Check sheet for the modelled part. Datum: model origin and axes. Units: mm. A direction names the side the tool comes from. Give positions to 0.01 mm unless a question says otherwise; leave off trailing zeros. Order: outer loops, then holes, each group sorted by start corner. A loop starts at its lowest first (then second) coordinate and runs counter-clockwise, first axis right, second up. Notation, with made-up numbers: M 63,28 L 97,28 A29 ccw 97,49 Z; hole C 79,15 d6. An arc over 180 degrees is marked long. One line per question, with ' | ' between items. Start each with the question number.
```python
from build123d import *

# Parameters (mm, degrees)
F1_DEPTH = 2
F2_R     = 2
F3_R     = 0.5


with BuildPart() as f1:
    # F0 (on Top) → F1 (new body)
    with BuildSketch(Plane.XY):
        with BuildLine():
            Line((2.5, 7.5), (2.5, 0))
            ThreePointArc((2.5, 0), (0, -2.5), (-2.5, 0))
            Line((-2.5, 0), (-2.5, 7.5))
            Line((-2.5, 7.5), (-7.5, 7.5))
            Line((-7.5, 7.5), (-7.5, -7.5))
            Line((-7.5, -7.5), (7.5, -7.5))
            Line((7.5, -7.5), (7.5, 7.5))
            Line((7.5, 7.5), (2.5, 7.5))
        make_face()
    extrude(amount=F1_DEPTH)

    # F2
    f2_edges = [f1.edges().sort_by_distance(p)[0] for p in [
        (7.5, -7.5, 1),
        (-7.5, -7.5, 1),
        (7.5, 7.5, 1),
        (2.5, 7.5, 1),
        (-2.5, 7.5, 1),
        (-7.5, 7.5, 1),
    ]]
    fillet(f2_edges, radius=F2_R)

    # F3
    f3_edges = [f1.edges().sort_by_distance(p)[0] for p in [
        (7.5, 0, 2),
        (6.914214, -6.914214, 2),
        (6.914214, 6.914214, 2),
        (0, -7.5, 2),
        (5, 7.5, 2),
        (-6.914214, -6.914214, 2),
        (3.085786, 6.914214, 2),
        (-7.5, 0, 2),
        (2.5, 2.75, 2),
        (-6.914214, 6.914214, 2),
        (0, -2.5, 2),
        (-5, 7.5, 2),
        (-2.5, 2.75, 2),
        (-3.085786, 6.914214, 2),
        (7.5, 0, 0),
        (6.914214, -6.914214, 0),
        (6.914214, 6.914214, 0),
        (0, -7.5, 0),
        (5, 7.5, 0),
        (-6.914214, -6.914214, 0),
        (3.085786, 6.914214, 0),
        (-7.5, 0, 0),
        (2.5, 2.75, 0),
        (-6.914214, 6.914214, 0),
        (0, -2.5, 0),
        (-5, 7.5, 0),
        (-2.5, 2.75, 0),
        (-3.085786, 6.914214, 0),
    ]]
    fillet(f3_edges, radius=F3_R)


solid = f1.part
```
Item 1: Section check A-A, the plane y = 3.75. Record the cut outline in (x, z), then the cut area to 3 significant figures.
Item 2: Scan lines: probe 1 along X at (y, z) = (3, 1.2); probe 2 along X at (y, z) = (-5.25, 1.55); probe 3 along X at (y, z) = (-0.75, 1.4). Record each from-to range of solid material in increasing order. Write a range as [from, to].
Item 3: Section check C-C, the plane z = 1.05. Record the cut outline in (x, y), then the cut area to 3 significant figures.
Item 4: Set-up check for faces 5 (the face through (-3.07, 6.9, 1.01)), 6 (the face through (7.5, 0, 1)): record each of +Z, -Z, +X, -X, +Y, -Y from which the full face is reachable in a straight line by a thin tool's end or side.
Item 5: Draft check along X on faces 1 (the face through (-2, -3, 0)), 2 (the face through (3.07, 6.9, 1.01)), 3 (the face through (-7.5, 0, 1)), 4 (the face through (6.9, -6.93, 1.01)). Enter one of: released by +X, released by -X, zero draft, split by the parting line, or undercut.
Item 6: Section check B-B, the plane x = 0. Record the cut outline in (y, z), then the cut area to 3 significant figures.
Reported:
1) outline: M -7.5,0.5 A0.5 ccw -7,0 L -3,0 A0.5 ccw -2.5,0.5 L -2.5,1.5 A0.5 ccw -3,2 L -7,2 A0.5 ccw -7.5,1.5 Z; M 2.5,0.5 A0.5 ccw 3,0 L 7,0 A0.5 ccw 7.5,0.5 L 7.5,1.5 A0.5 ccw 7,2 L 3,2 A0.5 ccw 2.5,1.5 Z | area: 19.6 mm^2
2) probe 1: x = [-7.5, -2.5], [2.5, 7.5] | probe 2: x = [-7.5, 7.5] | probe 3: x = [-7.5, -2.38], [2.38, 7.5]
3) outline: M -7.5,-5.5 A2 ccw -5.5,-7.5 L 5.5,-7.5 A2 ccw 7.5,-5.5 L 7.5,5.5 A2 ccw 5.5,7.5 L 4.5,7.5 A2 ccw 2.5,5.5 L 2.5,0 A2.5 cw -2.5,0 L -2.5,5.5 A2 ccw -4.5,7.5 L -5.5,7.5 A2 ccw -7.5,5.5 Z | area: 173 mm^2
4) face 5: +Z, -Z, +Y | face 6: +Z, -Z, +X, +Y, -Y
5) face 1: zero draft | face 2: undercut | face 3: released by -X | face 4: released by +X
6) outline: M -7.5,0.5 A0.5 ccw -7,0 L -3,0 A0.5 ccw -2.5,0.5 L -2.5,1.5 A0.5 ccw -3,2 L -7,2 A0.5 ccw -7.5,1.5 Z | area: 9.79 mm^2
